Read the model definition and answer for the solid it produces. Units are mm, in the model's axes. A direction names the side the tool comes from. Coordinates: 2 decimals unless noted, no trailing zeros. Write each loop counter-clockwise with the first axis right and the second up, starting at its lowest first coordinate (ties: lowest second). Pieces come first, ordered by that corner, then holes.
1) Find the intervals of material crossed by line 1 (Y direction, x = 2.8, z = -17.5); line 2 (Y direction, x = 19.5, z = 12); line 3 (Z direction, x = 20.25, y = 38.5), in increasing order.
2) Which of the six approach directions +Z, -Z, +X, -X, +Y, -Y give full straight-line access (tool end or side, diameter ignored) to faces 1 (the face through (17.444, -49.452, 23.566)), 2 (the face through (2, 15, 25))?
3) The part is cut by section B-B (x = 16). Give the number of separate pieces and of enclosed holes in the cut face, then the cut area to 3 significant figures.
4) The part is cut by section A-A (y = -15). Determine the outline of the cut face in (x, z), then the cut area to 3 significant figures.
5) Determine the mould class of faces 3 (the face through (21.5, 4, -46)), 4 (the face through (11, 1, -48.096)), 5 (the face through (17.444, -49.274, 36.923)) for opening direction Z: +Z half, -Z half, draft (parallel to the pull), parting line (faces both ways), or undercut.
6) The part is cut by section D-D (y = 34.5). Determine the outline of the cut face in (x, z), then the cut area to 3 significant figures.
7) The part is cut by section C-C (z = 36). Determine the outline of the cut face in (x, y).
8) Each of these flat-tipped pins is pushed along its axis until it touches: pin 1 Ø4.5 at (y, z) = (-47.5, -25.5) entering from +X; pin 2 Ø2.5 at (y, z) = (-47.5, 24) entering from +X. Where does it stop, or does it pass through?
from build123d import *

# Parameters (mm, degrees)
SKETCH_1_W                = 104
SKETCH_1_H                = 95.096423431
EXTRUDE_1_DEPTH           = 21.5
SKETCH_2_W                = 86
SKETCH_2_H                = 86
CUT_EXTRUDE_1_DEPTH       = 17.5
HOLE_WIZARD_4_0_4_1_D     = 4
HOLE_WIZARD_4_0_4_1_DEPTH = 8
HOLE_WIZARD_5_0_5_1_D     = 5
HOLE_WIZARD_5_0_5_1_DEPTH = 9
HOLE_WIZARD_5_0_5_2_D     = 5
HOLE_WIZARD_5_0_5_2_DEPTH = 21.5
HOLE_WIZARD_5_0_5_3_D     = 5
HOLE_WIZARD_5_0_5_3_DEPTH = 104
FILLET_1_R                = 2
FILLET_2_R                = 4


with BuildPart() as part:
    # 草图1 → 凸台-拉伸1 (new body)
    with BuildSketch(Plane(origin=(0, 0, 0), x_dir=(0, -1, 0), z_dir=(-1, 0, 0))):
        with Locations((0, -0.548211716)):
            Rectangle(SKETCH_1_W, SKETCH_1_H)
    extrude(amount=-EXTRUDE_1_DEPTH)

    # 草图2 → 切除-拉伸1 (cut)
    with BuildSketch(Plane(origin=(21.5, 0, 0), x_dir=(0, 0, -1), z_dir=(1, 0, 0))):
        Rectangle(SKETCH_2_W, SKETCH_2_H)
    extrude(amount=-CUT_EXTRUDE_1_DEPTH, mode=Mode.SUBTRACT)

    # Ø4.0 (4) 直径孔1
    with Locations(Plane(origin=(21.5, 0, 0), x_dir=(0, 0, -1), z_dir=(1, 0, 0))):
        with Locations((0, 47.5), (12, 47.5), (24, 47.5), (-12, 47.5), (-24, 47.5), (0, -47.5), (12, -47.5), (25.096423431, -47.5), (-12, -47.5), (-24, -47.5), (36, 47.5), (37.096423431, -47.5), (-36, -47.5), (-36, 47.5)):
            Hole(HOLE_WIZARD_4_0_4_1_D / 2, depth=HOLE_WIZARD_4_0_4_1_DEPTH)

    # Ø5.0 (5) 直径孔1
    with Locations(Plane(origin=(0, -52, 0), x_dir=(-1, 0, 0), z_dir=(0, -1, 0))):
        with Locations((-9.5, 15), (-9.5, -15)):
            Hole(HOLE_WIZARD_5_0_5_1_D / 2, depth=HOLE_WIZARD_5_0_5_1_DEPTH)

    # Ø5.0 (5) 直径孔2
    with Locations(Plane.ZY):
        with Locations((-17.5, -27.5), (-17.5, 27.5), (17.5, 27.5), (17.5, -27.5), (-22.5, -15), (-22.5, 15), (22.5, 15), (22.5, -15)):
            Hole(HOLE_WIZARD_5_0_5_2_D / 2, depth=HOLE_WIZARD_5_0_5_2_DEPTH)

    # Ø5.0 (5) 直径孔3
    with Locations(Plane(origin=(0, 52, 0), x_dir=(1, 0, 0), z_dir=(0, 1, 0))):
        with Locations((9.5, -15), (9.5, 15)):
            Hole(HOLE_WIZARD_5_0_5_3_D / 2, depth=HOLE_WIZARD_5_0_5_3_DEPTH)

    # 圆角1
    fillet_1_edges = [part.edges().sort_by_distance(p)[0] for p in [
        (12.75, -43, -43),
        (12.75, -43, 43),
        (12.75, 43, 43),
        (12.75, 43, -43),
    ]]
    fillet(fillet_1_edges, radius=FILLET_1_R)

    # 圆角2
    fillet_2_edges = [part.edges().sort_by_distance(p)[0] for p in [
        (10.75, -52, 47),
        (10.75, -52, -48.096423431),
        (10.75, 52, -48.096423431),
        (10.75, 52, 47),
    ]]
    fillet(fillet_2_edges, radius=FILLET_2_R)


solid = part.part
Reported:
1. line 1: y = -52 to -30, -25 to 25, 30 to 52
1. line 2: y = -52 to -49.5, -45.5 to -43, 43 to 45.5, 49.5 to 52
1. line 3: z = -48.1 to -43, 43 to 47
2. face 1: +X
2. face 2: +X, -X
3. separate pieces: 1
3. enclosed holes: 15
3. area: 2,310 mm2
4. outline: (0, -48.1) - (21.5, -48.1) - (21.5, -43) - (4, -43) - (4, -25) - (0, -25) - close; (0, -20) - (4, -20) - (4, 20) - (0, 20) - close; (0, 25) - (4, 25) - (4, 43) - (21.5, 43) - (21.5, 47) - (0, 47) - close
4. area: 500 mm2
5. face 3: draft
5. face 4: -Z half
5. face 5: undercut
6. outline: (0, -48.1) - (21.5, -48.1) - (21.5, -43) - (4, -43) - (4, 43) - (21.5, 43) - (21.5, 47) - (0, 47) - close
6. area: 540 mm2
7. outline: (0, -52) - (21.5, -52) - (21.5, -49.5) - (13.5, -49.5) - (13.5, -45.5) - (21.5, -45.5) - (21.5, -43) - (4, -43) - (4, 43) - (21.5, 43) - (21.5, 45.5) - (13.5, 45.5) - (13.5, 49.5) - (21.5, 49.5) - (21.5, 52) - (0, 52) - close
8. pin 1: stops at x = 21.5
8. pin 2: stops at x = 13.5
